Autodesk Inventor part; units mm, degrees
ref_plane "Start Plane" through (0, 0, 0) normal (1, 0, 0) x (0, 1, 0)
ref_plane "XZ Plane" through (0, 0, 0) normal (0, 1, 0) x (-1, 0, 0)
ref_plane "XY Plane" through (0, 0, 0) normal (0, 0, 1) x (1, 0, 0)
sketch "Main Sketch" plane through (0, 0, 0) normal (0, 0, 1) x (1, 0, 0)
  line L0 (0, 0) -> (45, 0)
  line L1 (0, 0) -> (0, 7.65)
  line L2 (45, 7.65) -> (45, 0)
  line L3 (0, 7.65) -> (45, 7.65)
  dimension "d3" = 15.3
revolve "Revolution1" add sketch "Main Sketch" angle 360 about axis through (0, 0, 0) along (1, 0, 0)
chamfer "Chamfer3" distance 0.5 angle 45 1 edges at (45, -7.65, 0) measured on face at (30, 7.5509, -1.2271)
chamfer "Chamfer2" distance 0.5 angle 45 1 edges at (0, -7.65, 0) measured on face at (14.8333, 7.6252, -0.6156)
properties part number "Eje silla - Interno" material "Steel"
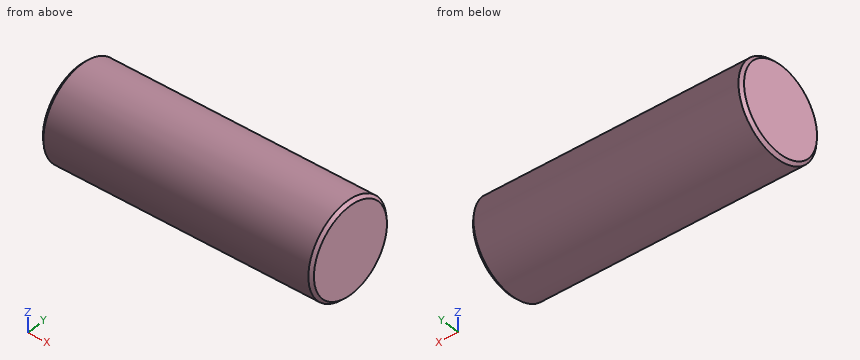
Can you work these out from the model? Positions are in its coordinate system, mm. Round coordinates to 2 decimals unless told otherwise and drop trailing zeros. Write each loop counter-clockwise with the first axis right and the second up, starting at its lowest first coordinate (ties: lowest second). Pieces come first, ordered by that corner, then holes. Notation, with made-up numbers: M -1,34.25 L 37,34.25 A20 ccw 37,47.25 Z; hole C -1.75,-5 d1. An arc over 180 degrees is marked long. Use a Markdown table: item, result.
Item 1: If I drill on line 1 along X through (y, z) = (-2.5, 6.75); line 2 along Y through (x, z) = (23, -5.25); line 3 along Z through (x, y) = (38.5, 4), over which ranges is the centre line in solid material (lowest first)? Write a range as [from, to].
Found:
| item | result |
|---|---|
| line 1 | x = [0.05, 44.95] |
| line 2 | y = [-5.56, 5.56] |
| line 3 | z = [-6.52, 6.52] |
Item 2: I want a section at A-A (x = 38). List the corners of the cut face in (y, z) for me, and give its area (3 significant figures).
Found:
| item | result |
|---|---|
| outline | C 0,0 d15.3 |
| area | 184 mm2 |
Item 3: For pin 1 Ø2 at (x, y) = (28.5, 5.5) entering from +Z; pin 2 Ø8 at (x, y) = (24, 6) entering from +Z; pin 3 Ø1 at (x, y) = (37, 4) entering from -Z; pin 4 Ø8 at (x, y) = (14.5, 1) entering from -Z, each with a flat end and sliding along its axis, tell me the tip position at first contact or that it passes through.
Found:
| item | result |
|---|---|
| pin 1 | stops at z = 6.19 |
| pin 2 | stops at z = 7.38 |
| pin 3 | stops at z = -6.8 |
| pin 4 | stops at z = -7.65 |
